Work out the finished part from the listing and answer in its coordinate system (mm). A direction names the side the tool comes from. Coordinates: 2 decimals unless noted, no trailing zeros. Loops run counter-clockwise (first coordinate to the right, second up) from the corner with the lowest first, then second, coordinate; pieces in that order, holes last. Notation, with made-up numbers: (53, -14) -> (73, -14) arc R22 ccw to (73, -5) -> close; hole circle Ø5 at (87.5, -24). An arc over 180 degrees is marked (long way). Answer as CSV lines item,"result".
```python
from build123d import *

# Parameters (mm, degrees)
F0_R     = 12.446
F1_DEPTH = 45.72
F3_W     = 33.02
F3_H     = 6.35
F4_DEPTH = 2.54
F5_R     = 11.0998
F6_DEPTH = 43.942
F7_W     = 5.7404
F7_H     = 13.462
F8_DEPTH = 25.4
F9_SIZE  = 1.27


with BuildPart() as f1:
    # F0 (on Top) → F1 (new body)
    with BuildSketch(Plane.XY):
        Circle(F0_R)
    extrude(amount=F1_DEPTH)

    # F3 (on offset) → F4 (join)
    with BuildSketch(Plane.XY.offset(5.461)):
        Rectangle(F3_W, F3_H)
    extrude(amount=F4_DEPTH)

    # F5 (on face) → F6 (cut)
    with BuildSketch(Plane.XY.offset(45.72)):
        Circle(F5_R)
    extrude(amount=-F6_DEPTH, mode=Mode.SUBTRACT)

    # F7 (on Front) → F8 (cut)
    with BuildSketch(Plane.XZ):
        with Locations((0, 8.509)):
            Rectangle(F7_W, F7_H)
    extrude(amount=-F8_DEPTH, mode=Mode.SUBTRACT)

    # F9
    f9_edges = [f1.edges().sort_by_distance(p)[0] for p in [
        (-12.446, 0, 0),
        (-16.51, 0, 8.001),
        (16.51, 0, 8.001),
        (-11.0998, 0, 45.72),
    ]]
    chamfer(f9_edges, length=F9_SIZE)


solid = f1.part
```
(1) A cutting plane is placed at D-D, the plane z = 11. Write down the section's boundary in (x, y), and give its area (3 significant figures).
Computed values:
outline,"(-2.87, 10.72) -> (-2.87, 12.11) arc R12.45 ccw (long way) to (2.87, 12.11) -> (2.87, 10.72) arc R11.1 cw (long way) to start"
area,"91.8 mm2"
(2) A cutting plane is placed at C-C, the plane z = 34.5. Write down the section's boundary in (x, y), and give its area (3 significant figures).
Computed values:
outline,"circle Ø24.89 at (0, 0); hole circle Ø22.2 at (0, 0)"
area,"99.6 mm2"
(3) Consider line 1 along Y through (x, z) = (0, 34); line 2 along Z through (x, y) = (-1.5, 3.75); line 3 along X through (y, z) = (4.75, 41). Determine where each line is inside the solid, lowest interval first.
Computed values:
line 1,"-12.45 to -11.1, 11.1 to 12.45"
line 2,"0 to 1.78"
line 3,"-11.5 to -10.03, 10.03 to 11.5"
(4) Which of the six approach directions +Z, -Z, +X, -X, +Y, -Y give full straight-line access (tool end or side, diameter ignored) to faces 1 (the face through (14, 3.175, 7)), 2 (the face through (-2.87, 11, 8)), 3 (the face through (14, -3.175, 7))?
Computed values:
face 1,"+Z, -Z, +X, +Y"
face 2,"+Y"
face 3,"+Z, -Z, +X, -Y"
(5) A cutting plane is placed at B-B, the plane y = 0. Write down the section's boundary in (x, z), and give its area (3 significant figures).
Computed values:
outline,"(-16.51, 5.46) -> (-12.45, 5.46) -> (-12.45, 1.27) -> (-11.18, 0) -> (11.18, 0) -> (12.45, 1.27) -> (12.45, 5.46) -> (16.51, 5.46) -> (16.51, 6.73) -> (15.24, 8) -> (12.45, 8) -> (12.45, 45.72) -> (12.37, 45.72) -> (11.1, 44.45) -> (11.1, 1.78) -> (-11.1, 1.78) -> (-11.1, 44.45) -> (-12.37, 45.72) -> (-12.45, 45.72) -> (-12.45, 8) -> (-15.24, 8) -> (-16.51, 6.73) -> close"
area,"178 mm2"
(6) Flat-ended cylindrical pins translate along their axes: pin 1 Ø0.8 at (x, z) = (-14.5, 6.5) entering from +Y (3 decimals); pin 2 Ø2 at (x, z) = (14, 6) entering from -Y (3 decimals); pin 3 Ø2 at (y, z) = (-7, 16.5) entering from +X. Find the tip coordinate at first contact, or state that the pin passes through.
Computed values:
pin 1,"y = 3.175"
pin 2,"y = -3.175"
pin 3,"x = 10.9"
(7) A cutting plane is placed at A-A, the plane x = 0. Write down the section's boundary in (y, z), and give its area (3 significant figures).
Computed values:
outline,"(-12.45, 1.27) -> (-11.18, 0) -> (11.18, 0) -> (12.45, 1.27) -> (12.45, 1.78) -> (-11.1, 1.78) -> (-11.1, 44.45) -> (-12.37, 45.72) -> (-12.45, 45.72) -> close; (11.1, 15.24) -> (12.45, 15.24) -> (12.45, 45.72) -> (12.37, 45.72) -> (11.1, 44.45) -> close"
area,"141 mm2"
(8) For a pull along X with two mould halves and no side action, classify faces 4 (the face through (-16.51, 0, 6)), 5 (the face through (-14, 0, 8.001)), 6 (the face through (5.12, -9.85, 23.41)), 7 (the face through (0, 12, 15.24)) as pulls with the +X half, pulls with the -X half, needs draft (parallel to the pull), parting line crosses it, or undercut.
Computed values:
face 4,"pulls with the -X half"
face 5,"needs draft"
face 6,"undercut"
face 7,"undercut"
